Check sheet for the modelled part. Datum: model origin and axes. Units: mm. Coordinates: 2 decimals unless noted, no trailing zeros. Write each loop counter-clockwise with the first axis right and the second up, starting at its lowest first coordinate (ties: lowest second). Pieces come first, ordered by that corner, then holes. Notation, with made-up numbers: M 87,22.5 L 123,22.5 A22 ccw 123,49.5 Z; hole C 89.5,-25.5 d9. An arc over 180 degrees is marked long. Answer as CSV lines item,"result".
from build123d import *

# Parameters (mm, degrees)
SKETCH1_W           = 88.9
SKETCH1_H           = 22.86
BOSS_EXTRUDE1_DEPTH = 5.2578
FILLET1_R           = 5.08
FILLET2_R           = 5.08
FILLET3_R           = 5.08
FILLET4_R           = 5.08


with BuildPart() as part:
    # Sketch1 → Boss-Extrude1 (new body)
    with BuildSketch(Plane.XY):
        Rectangle(SKETCH1_W, SKETCH1_H)
    extrude(amount=BOSS_EXTRUDE1_DEPTH)

    # Fillet1
    fillet1_edges = [part.edges().sort_by_distance(p)[0] for p in [
        (-44.45, 11.43, 2.6289),
    ]]
    fillet(fillet1_edges, radius=FILLET1_R)

    # Fillet2
    fillet2_edges = [part.edges().sort_by_distance(p)[0] for p in [
        (44.45, 11.43, 2.6289),
    ]]
    fillet(fillet2_edges, radius=FILLET2_R)

    # Fillet3
    fillet3_edges = [part.edges().sort_by_distance(p)[0] for p in [
        (44.45, -11.43, 2.6289),
    ]]
    fillet(fillet3_edges, radius=FILLET3_R)

    # Fillet4
    fillet4_edges = [part.edges().sort_by_distance(p)[0] for p in [
        (-44.45, -11.43, 2.6289),
    ]]
    fillet(fillet4_edges, radius=FILLET4_R)


solid = part.part
1) Thickness scan on line 1 along X through (y, z) = (6.5, 4.9); line 2 along X through (y, z) = (-7.75, 2.75). Record the ranges inside material, lowest first.
Answer key:
line 1,"x = -44.45 to 44.45"
line 2,"x = -44.25 to 44.25"
2) Depth check by flat-ended pin: P1, Ø1.5, axis at y = -8, z = 2, coming from the +X side. Enter the tip coordinate at first touch or a pass-through.
Answer key:
P1,"stops at x = 44.37"
3) Section check A-A, the plane y = -9. Record the boundary of the cut face in (x, z), plus the area to 3 significant figures.
Answer key:
outline,"M -43.7,0 L 43.7,0 L 43.7,5.26 L -43.7,5.26 Z"
area,"460 mm2"
